Input: part model. Units: mm. Frame: model coordinates. A direction names the side the tool comes from. Give positions to 0.01 mm unless a question says otherwise; leave off trailing zeros. Write each loop counter-clockwise with the first axis right and the second up, starting at its lowest first coordinate (ties: lowest second). Pieces come first, ordered by that corner, then holes. Notation, with made-up numbers: (79, 48) - (91, 48) arc R18 ccw to (91, 75) - close; hole circle Ø1 at (-36, 52.5). An arc over 180 degrees is marked (long way). Use a Markdown table: item, result. Add a question column.
1. Section query C-C, the plane x = 123.5. Return loops of the section in (y, z), plus the area to 3 significant figures.
2. Section query B-B, the plane z = 95.5. Return loops of the section in (x, y).
3. Mould query, pull axis Y, two halves, no side actions, for faces 6 (the cylindrical face through (9.7, -34.9, 216.2)), 7 (the flat face through (16, 78, 219.382)), 8 (the flat face through (16, -66.976, -14)). Classes: released by +Y, released by -Y, zero draft, split by the parting line, or undercut.
4. Section query A-A, the plane y = 67. Return loops of the section in (x, z), plus the area to 3 significant figures.
5. Material intervals for probe 1 along Z at (x, y) = (13, 184); probe 2 along Y at (x, z) = (8.5, 103.5), sorted ascending.
6. Set-up query: faces 1 (the flat face through (0, 258, -14)), 2 (the flat face through (95, -47.926, -241)), 3 (the flat face through (95, 266, 200.332)), 4 (the flat face through (173.8, -57, -241)), 5 (the flat face through (9, 256.874, -13)). Return all of +Z, -Z, +X, -X, +Y, -Y with unobstructed straight access to the full face (end or side cutting, diameter ignored); none if empty.
7. Pin query (flat end, axial travel): pin 1 (5.5 mm diameter, centred on y = -60.5, z = -28, fed in from +X). Return the tip coordinate at first contact, or that it passes through.
```python
from build123d import *

# Parameters (mm, degrees)
SKETCH2_W           = 431.8
SKETCH2_H           = 19.05
SKETCH2_W_2         = 19.05
SKETCH2_H_2         = 342.9
BOSS_EXTRUDE1_DEPTH = 19.05
SKETCH3_R           = 6.35
CUT_EXTRUDE1_DEPTH  = 25.4
SKETCH4_W           = 19.05
SKETCH4_H           = 19.05
BOSS_EXTRUDE2_DEPTH = 154.7495


with BuildPart() as part:
    # Sketch2 → Boss-Extrude1 (new body)
    with BuildSketch(Plane(origin=(0, 0, 0), x_dir=(0, 0, -1), z_dir=(1, 0, 0))):
        with Locations((15.568493322, 266.398734107)):
            Rectangle(SKETCH2_W, SKETCH2_H)
        with Locations((-209.856506678, 104.473734107)):
            Rectangle(SKETCH2_W_2, SKETCH2_H_2)
        with Locations((15.568493322, -57.451265893)):
            Rectangle(SKETCH2_W, SKETCH2_H)
        Polygon((250.518493322, 275.923734107), (231.468493322, 275.923734107), (231.468493322, 256.873734107), (231.468493322, -47.926265893), (231.468493322, -66.976265893), (250.518493322, -66.976265893), align=None)
    extrude(amount=BOSS_EXTRUDE1_DEPTH)

    # Sketch3 → Cut-Extrude1 (cut)
    with BuildSketch(Plane(origin=(19.05, 0, 0), x_dir=(0, 0, -1), z_dir=(1, 0, 0))):
        with Locations((-209.856506678, 15.573734107)):
            Circle(SKETCH3_R)
        with Locations((-209.856506678, -35.226265893)):
            Circle(SKETCH3_R)
        with Locations((240.993493322, -35.226265893)):
            Circle(SKETCH3_R)
        with Locations((240.993493322, 15.573734107)):
            Circle(SKETCH3_R)
    extrude(amount=-CUT_EXTRUDE1_DEPTH, mode=Mode.SUBTRACT)

    # Sketch4 → Boss-Extrude2 (add)
    with BuildSketch(Plane(origin=(19.05, 0, 0), x_dir=(0, 0, -1), z_dir=(1, 0, 0))):
        with Locations((-209.856506678, -57.451265893)):
            Rectangle(SKETCH4_W, SKETCH4_H)
        with Locations((-209.856506678, 266.398734107)):
            Rectangle(SKETCH4_W, SKETCH4_H)
        with Locations((240.993493322, 266.398734107)):
            Rectangle(SKETCH4_W, SKETCH4_H)
        with Locations((240.993493322, -57.451265893)):
            Rectangle(SKETCH4_W, SKETCH4_H)
    extrude(amount=BOSS_EXTRUDE2_DEPTH)


solid = part.part
```
Result sheet:
| question | item | result |
|---|---|---|
| 1 | outline | (-66.98, -250.52) - (-47.93, -250.52) - (-47.93, -231.47) - (-66.98, -231.47) - close; (-66.98, 200.33) - (-47.93, 200.33) - (-47.93, 219.38) - (-66.98, 219.38) - close; (256.87, -250.52) - (275.92, -250.52) - (275.92, -231.47) - (256.87, -231.47) - close; (256.87, 200.33) - (275.92, 200.33) - (275.92, 219.38) - (256.87, 219.38) - close |
| 1 | area | 1,450 mm² |
| 2 | outline | (0, -66.98) - (19.05, -66.98) - (19.05, -47.93) - (0, -47.93) - close; (0, 256.87) - (19.05, 256.87) - (19.05, 275.92) - (0, 275.92) - close |
| 3 | face 6 | undercut |
| 3 | face 7 | zero draft |
| 3 | face 8 | released by -Y |
| 4 | outline | (0, -250.52) - (19.05, -250.52) - (19.05, -231.47) - (0, -231.47) - close; (0, 200.33) - (19.05, 200.33) - (19.05, 219.38) - (0, 219.38) - close |
| 4 | area | 726 mm² |
| 5 | probe 1 | z = -250.52 to -231.47, 200.33 to 219.38 |
| 5 | probe 2 | y = -66.98 to -47.93, 256.87 to 275.92 |
| 6 | face 1 | +Z, -Z, -X, +Y, -Y |
| 6 | face 2 | +Z, -Z, +X |
| 6 | face 3 | +X, +Y, -Y |
| 6 | face 4 | +Z, -Z, +X, +Y, -Y |
| 6 | face 5 | +X, -X |
| 7 | pin 1 | stops at x = 19.05 |
